The figure shows three views and two pictorial views of one solid part (mm, origin at its lowest corner). Answer the questions. A direction names the side the tool comes from. Round coordinates to 2 decimals unless told otherwise and drop trailing zeros. Write each loop counter-clockwise with the first axis right and the second up, starting at its lowest first coordinate (ties: lowest second). Pieces come first, ordered by that corner, then holes.
Item 1: For a pull along X with two mould halves and no side action, classify the marked faces 1 and 2 as +X half, -X half, draft (parallel to the pull), parting line (faces both ways), or undercut.
Item 2: Find section A-A on x = 50. Give the vertices of the cut face in (y, z), then the cut area to 3 significant figures.
Item 3: Find section D-D on x = 3. Give the vertices of the cut face in (y, z).
Item 4: Each of these flat-tipped pins is pushed along its axis until it touches: pin 1 (1.5 mm diameter, centred on x = 42.5, y = 7.5, fed in from -Z); pin 2 (2.5 mm diameter, centred on x = 82, z = 3.5, fed in from +Y); pin 3 (1.5 mm diameter, centred on y = 7, z = 1.5, fed in from +X); pin 4 (2.5 mm diameter, centred on x = 78.5, z = 4, fed in from -Y). Where does it stop, or does it pass through?
Item 5: A tool of negligible diameter and unlimited length cuts with its end or side. For the marked faces 3, 4, 5 and 6, from which of +Z, -Z, +X, -X, +Y, -Y can it reach the whole face along a straight path? Write none if from no direction.
Item 6: Find section B-B on y = 3. Give the vertices of the cut face in (x, z), then the cut area to 3 significant figures.
Item 7: Find the intervals of material crossed by probe 1 along X at (y, z) = (14, 3.5); probe 2 along X at (y, z) = (3, 2.15); probe 3 along X at (y, z) = (2.5, 2.8), in increasing order.
Item 8: Find section C-C on y = 12.75. Give the vertices of the cut face in (x, z).
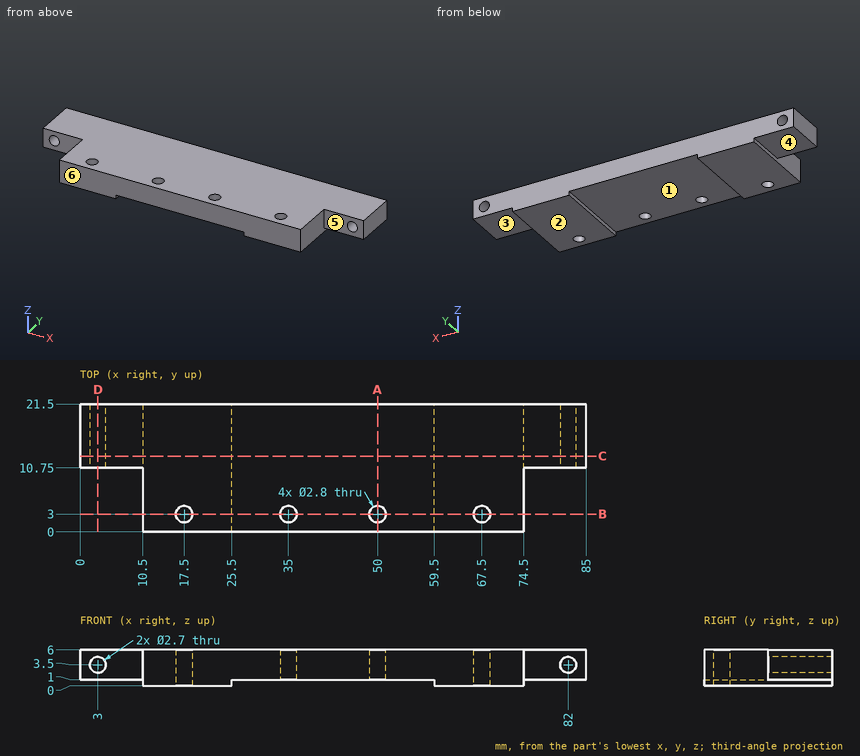
Check values:
1. face 1: undercut
1. face 2: draft
2. outline: (0, 1) - (1.6, 1) - (1.6, 6) - (0, 6) - close; (4.4, 1) - (21.5, 1) - (21.5, 6) - (4.4, 6) - close
2. area: 93.5 mm2
3. outline: (10.75, 1) - (21.5, 1) - (21.5, 2.15) - (10.75, 2.15) - close; (10.75, 4.85) - (21.5, 4.85) - (21.5, 6) - (10.75, 6) - close
4. pin 1: stops at z = 1
4. pin 2: passes through
4. pin 3: stops at x = 74.5
4. pin 4: stops at y = 10.75
5. face 3: -Z, +X, +Y, -Y
5. face 4: -Z, -X, +Y, -Y
5. face 5: +Z, -Z, +X, -Y
5. face 6: +Z, -Z, +X, -X, -Y
6. outline: (10.5, 0) - (16.1, 0) - (16.1, 6) - (10.5, 6) - close; (18.9, 0) - (25.5, 0) - (25.5, 1) - (33.6, 1) - (33.6, 6) - (18.9, 6) - close; (36.4, 1) - (48.6, 1) - (48.6, 6) - (36.4, 6) - close; (51.4, 1) - (59.5, 1) - (59.5, 0) - (66.1, 0) - (66.1, 6) - (51.4, 6) - close; (68.9, 0) - (74.5, 0) - (74.5, 6) - (68.9, 6) - close
6. area: 288 mm2
7. probe 1: x = 0 to 1.65, 4.35 to 80.65, 83.35 to 85
7. probe 2: x = 10.5 to 16.1, 18.9 to 33.6, 36.4 to 48.6, 51.4 to 66.1, 68.9 to 74.5
7. probe 3: x = 10.5 to 16.19, 18.81 to 33.69, 36.31 to 48.69, 51.31 to 66.19, 68.81 to 74.5
8. outline: (0, 1) - (10.5, 1) - (10.5, 0) - (25.5, 0) - (25.5, 1) - (59.5, 1) - (59.5, 0) - (74.5, 0) - (74.5, 1) - (85, 1) - (85, 6) - (0, 6) - close; hole circle Ø2.7 at (3, 3.5); hole circle Ø2.7 at (82, 3.5)
